Model file for the job. Use its own axes, mm. Face numbers are marked on the shaded views. A direction names the side the tool comes from. Coordinates: 2 decimals unless noted, no trailing zeros. Loops run counter-clockwise (first coordinate to the right, second up) from the corner with the lowest first, then second, coordinate; pieces in that order, holes last. Notation, with made-up numbers: (19.25, 34) -> (74.25, 34) arc R28 ccw to (74.25, 69) -> close; hole circle Ø8 at (-2.5, 54). An arc over 180 degrees is marked (long way). Use one line per item in the form item = value.
```python
from build123d import *

# Parameters (mm, degrees)
MAIN_DEPTH            = 27.5
SERVOSQUAREHOLE_DEPTH = 37.962819157
SKETCH2_R             = 1.5
SKETCH2_R_2           = 1.25
FIXINGHOLE_DEPTH      = 37.962819157
FILLET1_R             = 1
SKETCH4_W             = 6
SKETCH4_H             = 22.5
CUT_EXTRUDE2_DEPTH    = 37.962819157
FILLET2_R             = 10


with BuildPart() as part:
    # Sketch1 → Main (new, symmetric)
    with BuildSketch(Plane.XY):
        Polygon((10, 0), (10, 8), (-23, 8), (-23, 2.706273437), (0, 2.706273437), (0, 0), (3.55, 0), (3.55, -1), (6.45, -1), (6.45, 0), align=None)
    extrude(amount=MAIN_DEPTH, both=True)

    # Sketch3 → ServoSquareHole (cut, through all)
    with BuildSketch(Plane(origin=(0, 8, 0), x_dir=(1, 0, 0), z_dir=(0, 1, 0))):
        Polygon((-20.5, 20.5), (-13.25, 20.5), (-13.25, 24.5), (-7.25, 24.5), (-7.25, 20.5), (0, 20.5), (0, -20.5), (-7.25, -20.5), (-7.25, -24.5), (-13.25, -24.5), (-13.25, -20.5), (-20.5, -20.5), align=None)
    extrude(amount=-SERVOSQUAREHOLE_DEPTH, mode=Mode.SUBTRACT)

    # Sketch2 → FixingHole (cut, through all)
    with BuildSketch(Plane(origin=(0, 8, 0), x_dir=(1, 0, 0), z_dir=(0, 1, 0))):
        with Locations(Location((5, 0, 0), (0, 0, 180))):
            Circle(SKETCH2_R)
        with Locations(Location((-15.25, 24.5, 0), (0, 0, 180))):
            Circle(SKETCH2_R_2)
        with Locations(Location((-15.25, -24.5, 0), (0, 0, 180))):
            Circle(SKETCH2_R_2)
        with Locations(Location((-5.25, 24.5, 0), (0, 0, 180))):
            Circle(SKETCH2_R_2)
        with Locations(Location((-5.25, -24.5, 0), (0, 0, 180))):
            Circle(SKETCH2_R_2)
    extrude(amount=-FIXINGHOLE_DEPTH, mode=Mode.SUBTRACT)

    # Fillet1
    fillet1_edges = [part.edges().sort_by_distance(p)[0] for p in [
        (-13.25, 5.353136719, -24.5),
        (-7.25, 5.353136719, -24.5),
        (-7.25, 5.353136719, 24.5),
        (-13.25, 5.353136719, 24.5),
    ]]
    fillet(fillet1_edges, radius=FILLET1_R)

    # Sketch4 → Cut-Extrude2 (cut, through all)
    with BuildSketch(Plane(origin=(0, 8, 0), x_dir=(1, 0, 0), z_dir=(0, 1, 0))):
        with Locations((7, 16.25)):
            Rectangle(SKETCH4_W, SKETCH4_H)
        with Locations((7, -16.25)):
            Rectangle(SKETCH4_W, SKETCH4_H)
    extrude(amount=-CUT_EXTRUDE2_DEPTH, mode=Mode.SUBTRACT)

    # Fillet2
    # the kernel refuses this fillet: 10 mm, written as the material it adds along each edge
    with BuildSketch(Plane(origin=(4, 8, 5), x_dir=(1, 0, 0), z_dir=(0, -1, 0))) as fillet2_piece_1_section:
        with BuildLine():
            CenterArc((10, 9.16515139), FILLET2_R, 180, 66.421821522)
            Line((0, 9.16515139), (-0.2, 9.16515139))
            Line((-0.2, 9.16515139), (-0.2, 0))
            Line((-0.2, 0), (0, -0.2))
            ThreePointArc((0, -0.2), (3, -0.2), (5.92, -0.183303028))
            Line((5.92, -0.183303028), (6, 0))
        make_face()
    fillet2_piece_1 = extrude(amount=9, mode=Mode.PRIVATE)
    fillet2_piece_1 = split(fillet2_piece_1, bisect_by=Plane(origin=(7.630084013, 0, 5.669805071), z_dir=(0, 1, 0)), keep=Keep.TOP, mode=Mode.PRIVATE)
    fillet2_piece_1 = split(fillet2_piece_1, bisect_by=Plane(origin=(6.45, 4, 5.669805071), z_dir=(1, 0, 0)), keep=Keep.TOP, mode=Mode.PRIVATE)
    add(fillet2_piece_1)
    with BuildSketch(Plane(origin=(4, 8, 5), x_dir=(1, 0, 0), z_dir=(0, -1, 0))) as fillet2_piece_2_section:
        with BuildLine():
            CenterArc((10, 9.16515139), FILLET2_R, 180, 66.421821522)
            Line((0, 9.16515139), (-0.2, 9.16515139))
            Line((-0.2, 9.16515139), (-0.2, 0))
            Line((-0.2, 0), (0, -0.2))
            ThreePointArc((0, -0.2), (3, -0.2), (5.92, -0.183303028))
            Line((5.92, -0.183303028), (6, 0))
        make_face()
    fillet2_piece_2 = extrude(amount=9, mode=Mode.PRIVATE)
    fillet2_piece_2 = split(fillet2_piece_2, bisect_by=Plane(origin=(4.860609572, 0, 7.751217471), z_dir=(0, 1, 0)), keep=Keep.TOP, mode=Mode.PRIVATE)
    fillet2_piece_2 = split(fillet2_piece_2, bisect_by=Plane(origin=(6.45, 4, 7.751217471), z_dir=(-1, 0, 0)), keep=Keep.TOP, mode=Mode.PRIVATE)
    add(fillet2_piece_2)
    with BuildSketch(Plane(origin=(4, 8, 5), x_dir=(1, 0, 0), z_dir=(0, -1, 0))) as fillet2_piece_3_section:
        with BuildLine():
            CenterArc((10, 9.16515139), FILLET2_R, 180, 66.421821522)
            Line((0, 9.16515139), (-0.2, 9.16515139))
            Line((-0.2, 9.16515139), (-0.2, 0))
            Line((-0.2, 0), (0, -0.2))
            ThreePointArc((0, -0.2), (3, -0.2), (5.92, -0.183303028))
            Line((5.92, -0.183303028), (6, 0))
        make_face()
    fillet2_piece_3 = extrude(amount=9, mode=Mode.PRIVATE)
    fillet2_piece_3 = split(fillet2_piece_3, bisect_by=Plane(origin=(4.860609572, 0, 7.751217471), z_dir=(0, -1, 0)), keep=Keep.TOP, mode=Mode.PRIVATE)
    fillet2_piece_3 = split(fillet2_piece_3, bisect_by=Plane(origin=(6.45, -0.5, 7.751217471), z_dir=(-1, 0, 0)), keep=Keep.TOP, mode=Mode.PRIVATE)
    add(fillet2_piece_3)
    with BuildSketch(Plane(origin=(4, 8, -5), x_dir=(0, 0, -1), z_dir=(0, -1, 0))) as fillet2_piece_4_section:
        with BuildLine():
            CenterArc((9.16515139, 10), FILLET2_R, 203.578178478, 66.421821522)
            Line((0, 6), (-0.183303028, 5.92))
            ThreePointArc((-0.183303028, 5.92), (-0.2, 3), (-0.2, 0))
            Line((-0.2, 0), (0, -0.2))
            Line((0, -0.2), (9.16515139, -0.2))
            Line((9.16515139, -0.2), (9.16515139, 0))
        make_face()
    fillet2_piece_4 = extrude(amount=9, mode=Mode.PRIVATE)
    fillet2_piece_4 = split(fillet2_piece_4, bisect_by=Plane(origin=(6.45, 4, -7.751217471), z_dir=(-1, 0, 0)), keep=Keep.TOP, mode=Mode.PRIVATE)
    fillet2_piece_4 = split(fillet2_piece_4, bisect_by=Plane(origin=(4.860609572, 0, -7.751217471), z_dir=(0, 1, 0)), keep=Keep.TOP, mode=Mode.PRIVATE)
    add(fillet2_piece_4)
    with BuildSketch(Plane(origin=(4, 8, -5), x_dir=(0, 0, -1), z_dir=(0, -1, 0))) as fillet2_piece_5_section:
        with BuildLine():
            CenterArc((9.16515139, 10), FILLET2_R, 203.578178478, 66.421821522)
            Line((0, 6), (-0.183303028, 5.92))
            ThreePointArc((-0.183303028, 5.92), (-0.2, 3), (-0.2, 0))
            Line((-0.2, 0), (0, -0.2))
            Line((0, -0.2), (9.16515139, -0.2))
            Line((9.16515139, -0.2), (9.16515139, 0))
        make_face()
    fillet2_piece_5 = extrude(amount=9, mode=Mode.PRIVATE)
    fillet2_piece_5 = split(fillet2_piece_5, bisect_by=Plane(origin=(6.45, 4, -5.669805071), z_dir=(1, 0, 0)), keep=Keep.TOP, mode=Mode.PRIVATE)
    fillet2_piece_5 = split(fillet2_piece_5, bisect_by=Plane(origin=(7.630084013, 0, -5.669805071), z_dir=(0, 1, 0)), keep=Keep.TOP, mode=Mode.PRIVATE)
    add(fillet2_piece_5)
    with BuildSketch(Plane(origin=(4, 8, -5), x_dir=(0, 0, -1), z_dir=(0, -1, 0))) as fillet2_piece_6_section:
        with BuildLine():
            CenterArc((9.16515139, 10), FILLET2_R, 203.578178478, 66.421821522)
            Line((0, 6), (-0.183303028, 5.92))
            ThreePointArc((-0.183303028, 5.92), (-0.2, 3), (-0.2, 0))
            Line((-0.2, 0), (0, -0.2))
            Line((0, -0.2), (9.16515139, -0.2))
            Line((9.16515139, -0.2), (9.16515139, 0))
        make_face()
    fillet2_piece_6 = extrude(amount=9, mode=Mode.PRIVATE)
    fillet2_piece_6 = split(fillet2_piece_6, bisect_by=Plane(origin=(6.45, -0.5, -7.751217471), z_dir=(-1, 0, 0)), keep=Keep.TOP, mode=Mode.PRIVATE)
    fillet2_piece_6 = split(fillet2_piece_6, bisect_by=Plane(origin=(4.860609572, 0, -7.751217471), z_dir=(0, -1, 0)), keep=Keep.TOP, mode=Mode.PRIVATE)
    add(fillet2_piece_6)


solid = part.part
```
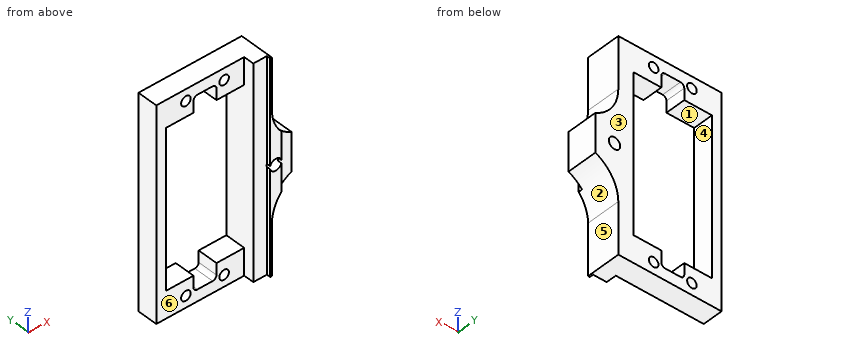
Q1. Mould opens along Z. For the marked faces 1, 2 and 3 say: released by +Z, released by -Z, zero draft, split by the parting line, or undercut.
Result:
face_1 = undercut
face_2 = released by -Z
face_3 = zero draft
Q2. Band-saw the part on A-A, the plane z = 21.5. Write the cut outline in (x, y), and give its area (3 significant figures).
Result:
outline = (-23, 2.71) -> (-13.25, 2.71) -> (-13.25, 8) -> (-23, 8) -> close; (-7.25, 2.71) -> (0, 2.71) -> (0, 0) -> (3.55, 0) -> (3.55, -1) -> (4, -1) -> (4, 8) -> (-7.25, 8) -> close
area = 122 mm2
Q3. Band-saw the part on C-C, the plane x = -15.25. Write the cut outline in (y, z).
Result:
outline = (2.71, -27.5) -> (8, -27.5) -> (8, -25.75) -> (2.71, -25.75) -> close; (2.71, -23.25) -> (8, -23.25) -> (8, -20.5) -> (2.71, -20.5) -> close; (2.71, 20.5) -> (8, 20.5) -> (8, 23.25) -> (2.71, 23.25) -> close; (2.71, 25.75) -> (8, 25.75) -> (8, 27.5) -> (2.71, 27.5) -> close
Q4. Pin check, flat tips, straight feed: pin 1 Ø1 at (y, z) = (2, -0.5) entering from -X; pin 2 Ø0.8 at (y, z) = (-0.5, -4) entering from +X; pin 3 Ø2.5 at (y, z) = (5.5, 9.5) entering from +X. Stop position of each tip, or through.
Result:
pin_1 = 0
pin_2 = 6.45
pin_3 = 5.94
Q5. Band-saw the part on D-D, the plane y = 6.5. State how many separate pieces and enclosed holes the cut face has, and give its area (3 significant figures).
Result:
separate_pieces = 1
enclosed_holes = 6
area = 661 mm2
Q6. Band-saw the part on B-B, the plane x = -10. Write the cut outline in (y, z).
Result:
outline = (2.71, -27.5) -> (8, -27.5) -> (8, -24.5) -> (2.71, -24.5) -> close; (2.71, 24.5) -> (8, 24.5) -> (8, 27.5) -> (2.71, 27.5) -> close
Q7. Which spindle directions (+Z, -Z, +X, -X, +Y, -Y) get a long thin tool onto all of the face, cutting with end or side? Do the marked faces 4, 5 and 6. Say none if no direction does.
Result:
face_4 = +Y, -Y
face_5 = -Z, +X, +Y, -Y
face_6 = +Z, -Z, -X, -Y
Q8. Wall check: line 1 along Z through (x, y) = (-15.25, 6.8); line 2 along X through (y, z) = (4, 0); line 3 along X through (y, z) = (3, 14.5). Give the ranges that are in metal, low to high.
Result:
line_1 = -27.5 to -25.75, -23.25 to -20.5, 20.5 to 23.25, 25.75 to 27.5
line_2 = -23 to -20.5, 0 to 3.5, 6.5 to 10
line_3 = -23 to -20.5, 0 to 4
